from build123d import *

# Parameters (mm, degrees)
BOSS_EXTRUDE1_DEPTH = 1000
SHELL1_T            = -15
BOSS_EXTRUDE2_DEPTH = 10
BOSS_EXTRUDE3_DEPTH = 15
BOSS_EXTRUDE4_DEPTH = 450
BOSS_EXTRUDE7_DEPTH = 450
BOSS_EXTRUDE8_DEPTH = 400
FILLET3_R           = 10


# Read off the part's stored shape, not the designer's step: Boss-Extrude3
with BuildPart() as part:
    # Sketch1 → Boss-Extrude1 (new body)
    with BuildSketch(Plane(origin=(0, 0, 0), x_dir=(1, 0, 0), z_dir=(0, 1, 0))):
        with BuildLine():
            Line((-200, -200), (200, -200))
            ThreePointArc((200, -200), (235.355339059, -185.355339059), (250, -150))
            Line((250, -150), (250, 150))
            ThreePointArc((250, 150), (235.355339059, 185.355339059), (200, 200))
            Line((200, 200), (-200, 200))
            ThreePointArc((-200, 200), (-235.355339059, 185.355339059), (-250, 150))
            Line((-250, 150), (-250, -150))
            ThreePointArc((-250, -150), (-235.355339059, -185.355339059), (-200, -200))
        make_face()
    extrude(amount=BOSS_EXTRUDE1_DEPTH)

    # Shell1
    shell1_openings = [part.faces().sort_by_distance(p)[0] for p in [
        (0, 1000, 0),
    ]]
    offset(amount=SHELL1_T, openings=shell1_openings, kind=Kind.INTERSECTION)

    # Sketch3 → Boss-Extrude2 (add)
    with BuildSketch(Plane(origin=(0, 1000, 0), x_dir=(1, 0, 0), z_dir=(0, 1, 0))):
        with BuildLine():
            Line((200, 0), (200, 100))
            Line((200, 100), (-200, 100))
            Line((-200, 100), (-200, 0))
            Line((-200, 0), (-250, 0))
            Line((-250, 0), (-250, -150))
            ThreePointArc((-250, -150), (-235.355339059, -185.355339059), (-200, -200))
            Line((-200, -200), (200, -200))
            ThreePointArc((200, -200), (235.355339059, -185.355339059), (250, -150))
            Line((250, -150), (250, 0))
            Line((250, 0), (200, 0))
        make_face()
    extrude(amount=BOSS_EXTRUDE2_DEPTH)

    # Boss-Extrude3 outline → Boss-Extrude3 (add)
    with BuildSketch(Plane(origin=(0, 1000, 0), x_dir=(1, 0, 0), z_dir=(0, 1, 0))):
        with BuildLine():
            Line((200, 100), (200, -100))
            ThreePointArc((200, -100), (185.355339059, -135.355339059), (150, -150))
            Line((150, -150), (-150, -150))
            ThreePointArc((-150, -150), (-185.355339059, -135.355339059), (-200, -100))
            Line((-200, -100), (-200, 100))
            ThreePointArc((-200, 100), (-199.74680765, 105.0254481), (-198.989794856, 110))
            Line((-198.989794856, 110), (-225, 110))
            Line((-225, 110), (-225, 0))
            Line((-225, 0), (-250, 0))
            Line((-250, 0), (-250, -150))
            ThreePointArc((-250, -150), (-235.355339059, -185.355339059), (-200, -200))
            Line((-200, -200), (200, -200))
            ThreePointArc((200, -200), (235.355339059, -185.355339059), (250, -150))
            Line((250, -150), (250, 0))
            Line((250, 0), (225, 0))
            Line((225, 0), (225, 110))
            Line((225, 110), (198.989794856, 110))
            ThreePointArc((198.989794856, 110), (199.74680765, 105.0254481), (200, 100))
        make_face()
    extrude(amount=BOSS_EXTRUDE3_DEPTH)

    # Sketch3<5> → Boss-Extrude4 (add)
    with BuildSketch(Plane(origin=(0, 1000, 0), x_dir=(1, 0, 0), z_dir=(0, 1, 0))):
        with BuildLine():
            Line((-250, 0), (-225, 0))
            Line((-225, 0), (-225, 100))
            Line((-225, 100), (-225, 110))
            Line((-225, 110), (-225, 125))
            ThreePointArc((-225, 125), (-210.355339059, 160.355339059), (-175, 175))
            Line((-175, 175), (175, 175))
            ThreePointArc((175, 175), (210.355339059, 160.355339059), (225, 125))
            Line((225, 125), (225, 110))
            Line((225, 110), (225, 100))
            Line((225, 100), (225, 0))
            Line((225, 0), (250, 0))
            Line((250, 0), (250, 150))
            ThreePointArc((250, 150), (235.355339059, 185.355339059), (200, 200))
            Line((200, 200), (-200, 200))
            ThreePointArc((-200, 200), (-235.355339059, 185.355339059), (-250, 150))
            Line((-250, 150), (-250, 0))
        make_face()
    extrude(amount=BOSS_EXTRUDE4_DEPTH)

    # Sketch3<7> → Boss-Extrude7 (add)
    with BuildSketch(Plane(origin=(0, 1000, 0), x_dir=(1, 0, 0), z_dir=(0, 1, 0))):
        with BuildLine():
            ThreePointArc((-198.989794856, 110), (-199.74680765, 105.0254481), (-200, 100))
            Line((-200, 100), (200, 100))
            ThreePointArc((200, 100), (199.74680765, 105.0254481), (198.989794856, 110))
            Line((198.989794856, 110), (-198.989794856, 110))
        make_face()
        with BuildLine():
            ThreePointArc((198.989794856, 110), (199.74680765, 105.0254481), (200, 100))
            Line((200, 100), (225, 100))
            Line((225, 100), (225, 110))
            Line((225, 110), (198.989794856, 110))
        make_face()
        with BuildLine():
            Line((-225, 100), (-200, 100))
            ThreePointArc((-200, 100), (-199.74680765, 105.0254481), (-198.989794856, 110))
            Line((-198.989794856, 110), (-225, 110))
            Line((-225, 110), (-225, 100))
        make_face()
    extrude(amount=BOSS_EXTRUDE7_DEPTH)

    # Sketch5 → Boss-Extrude8 (add)
    with BuildSketch(Plane(origin=(0, 1450, 0), x_dir=(1, 0, 0), z_dir=(0, 1, 0))):
        with BuildLine():
            Line((-200, -200), (200, -200))
            ThreePointArc((200, -200), (235.355339059, -185.355339059), (250, -150))
            Line((250, -150), (250, 150))
            ThreePointArc((250, 150), (235.355339059, 185.355339059), (200, 200))
            Line((200, 200), (-200, 200))
            ThreePointArc((-200, 200), (-235.355339059, 185.355339059), (-250, 150))
            Line((-250, 150), (-250, -150))
            ThreePointArc((-250, -150), (-235.355339059, -185.355339059), (-200, -200))
        make_face()
    extrude(amount=BOSS_EXTRUDE8_DEPTH)

    # Fillet3
    fillet3_edges = [part.edges().sort_by_distance(p)[0] for p in [
        (-225, 1232.5, 0),
        (225, 1450, -50),
        (237.5, 1450, 0),
        (225, 1232.5, 0),
        (-237.5, 1450, 0),
        (-250, 1232.5, 0),
        (250, 1232.5, 0),
        (-225, 1450, -50),
        (0, 1450, -100),
        (-235.355339059, 1450, 185.355339059),
        (0, 1450, 200),
        (235.355339059, 1450, 185.355339059),
        (250, 1450, 75),
        (-250, 1450, 75),
        (-237.5, 1015, 0),
        (0, 1015, 200),
        (250, 1015, 75),
        (237.5, 1015, 0),
        (225, 1015, -50),
        (235.355339059, 1015, 185.355339059),
        (-250, 1015, 75),
        (-235.355339059, 1015, 185.355339059),
        (-225, 1015, -50),
    ]]
    fillet(fillet3_edges, radius=FILLET3_R)


solid = part.part
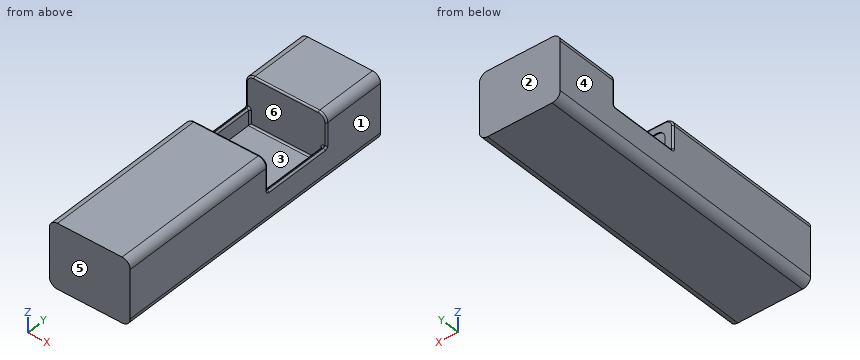
Design review of the part built by this model. Coordinates are the model's own, in mm. Face numbers are marked on the shaded views. A direction names the side the tool comes from. Round coordinates to 2 decimals unless told otherwise and drop trailing zeros. Loops run counter-clockwise (first coordinate to the right, second up) from the corner with the lowest first, then second, coordinate; pieces in that order, holes last. Notation, with made-up numbers: M 64,74.5 L 95,74.5 A22 ccw 95,107.5 Z; hole C 28,-26.5 d9. An arc over 180 degrees is marked long. Answer as a JSON object with one key per item and string values.
Item 1: Clearance check with flat-ended pins moving along their axes: P1, Ø2, axis at x = -3, z = -90, coming from the -Y side; P2, Ø5.5, axis at y = 1011.5, z = 34, coming from the +X side; P3, Ø12, axis at y = 902.5, z = 159, coming from the -X side. State where each tip first meets the part, or that it passes through.
Answer sheet:
{"P1": "stops at y = 0", "P2": "stops at x = 249.27", "P3": "stops at x = -249.91"}
Item 2: The part is to be moulded in two halves that separate along X. For the marked faces 1, 2, 3 and 4, say which applies: pulls with the +X half, pulls with the -X half, needs draft (parallel to the pull), parting line crosses it, or undercut.
Answer sheet:
{"face 1": "pulls with the +X half", "face 2": "needs draft", "face 3": "undercut", "face 4": "pulls with the -X half"}
Item 3: Wall thickness on L1, parallel to Y at x = -201.5, z = 75; L2, parallel to Y at x = 118.5, z = -66.5; L3, parallel to Z at x = 153, y = 1334.5: over which ranges is each line inside the solid? List them lowest first. Write a range as from..to.
Answer sheet:
{"L1": "y = 0..15, 1000..1015, 1450..1850", "L2": "y = 0..15, 1000..1010, 1450..1850", "L3": "z = -200..-175, -110..-100"}
Item 4: We need section C-C on x = -16. Give the boundary of the cut face in (y, z), and give its area (3 significant figures).
Answer sheet:
{"outline": "M 0,-200 L 1850,-200 L 1850,200 L 1460,200 A10 ccw 1450,190 L 1450,-90 A10 cw 1440,-100 L 1010,-100 L 1010,150 L 1015,150 L 1015,190 A10 ccw 1005,200 L 0,200 Z; hole M 15,-185 L 1000,-185 L 1000,-175 L 1450,-175 L 1450,-110 L 1000,-110 L 1000,185 L 15,185 Z", "area": "215,000 mm^2"}
Item 5: We need section B-B on y = 349. Give the boundary of the cut face in (x, z).
Answer sheet:
{"outline": "M -250,-150 A50 ccw -200,-200 L 200,-200 A50 ccw 250,-150 L 250,150 A50 ccw 200,200 L -200,200 A50 ccw -250,150 Z; hole M -235,-150 A35 ccw -200,-185 L 200,-185 A35 ccw 235,-150 L 235,150 A35 ccw 200,185 L -200,185 A35 ccw -235,150 Z"}
Item 6: Machinability: for the marked faces 5 and 6, which of the approach directions +Z, -Z, +X, -X, +Y, -Y give a long, thin tool a straight path to every point of the face, cutting with its end or side? Answer none if there is none.
Answer sheet:
{"face 5": "+Z, -Z, +X, -X, -Y", "face 6": "+Z"}
Item 7: We need section D-D on y = 1309. Give the boundary of the cut face in (x, z).
Answer sheet:
{"outline": "M -250,-150 A50 ccw -200,-200 L 200,-200 A50 ccw 250,-150 L 250,-10 A10 ccw 240,0 L 235,0 A10 ccw 225,-10 L 225,-100 L -225,-100 L -225,-10 A10 ccw -235,0 L -240,0 A10 ccw -250,-10 Z; hole M -225,-125 A50 ccw -175,-175 L 175,-175 A50 ccw 225,-125 L 225,-110 L -225,-110 Z"}
Item 8: We need section A-A on z = 27. Give the boundary of the cut face in (x, y).
Answer sheet:
{"outline": "M -250,0 L 250,0 L 250,1005 A10 ccw 240,1015 L 200,1015 L 200,1010 L -200,1010 L -200,1015 L -240,1015 A10 ccw -250,1005 Z; M -250,1460 A10 ccw -240,1450 L 240,1450 A10 ccw 250,1460 L 250,1850 L -250,1850 Z; hole M -235,15 L 235,15 L 235,1000 L -235,1000 Z"}
